Part print with two shaded views. Sizes in mm from the minimum x, y, z corner. A direction names the side the tool comes from. Give positions to 0.01 mm unless a question says otherwise; leave off trailing zeros. Write each loop counter-clockwise with the first axis right and the second up, starting at its lowest first coordinate (ties: lowest second). Pieces come first, ordered by that corner, then holes. Notation, with made-up numbers: (66, 7) - (103, 7) arc R26 cw to (103, 23) - close; hole circle Ø3 at (1.25, 86). An arc over 180 degrees is marked (long way). One line per item, written item: value. Start each with the question number.
(1) Cut at D-D, the plane y = 9.25. List the corners of the cut face in (x, z).
(2) Cut at B-B, the plane z = 19. State how many separate pieces and enclosed holes the cut face has.
(3) Cut at A-A, the plane x = 3.6. List the corners of the cut face in (y, z).
(4) Probe L1, parallel to Z at x = 21, y = 10; L2, parallel to Y at x = 29.6, z = 15; L3, parallel to X at y = 3, z = 11.75. List the from-to ranges inside material, lowest first.
(5) Cut at C-C, the plane y = 3.5. List the corners of the cut face in (x, z), and give its area (3 significant figures).
(6) Drop flat-ended pins along their axis: P1, Ø4.5, axis at x = 16.5, y = 12, coming from the -Z side; P2, Ø1, axis at x = 18, z = 9, coming from the +Y side (1 decimal); P3, Ø12.5, axis at x = 23, z = 10.5, coming from the +Y side. Give the stop position or say it passes through.
(7) 3-axis set-ups, long thin cutter, end or side, ignore diameter. For the marked faces 1 and 2: which of +Z, -Z, +X, -X, +Y, -Y reach the whole face in a straight line?
(8) Mould opens along Z. For the marked faces 3, 4 and 5 say: pulls with the +Z half, pulls with the -Z half, needs draft (parallel to the pull), parting line crosses it, or undercut.
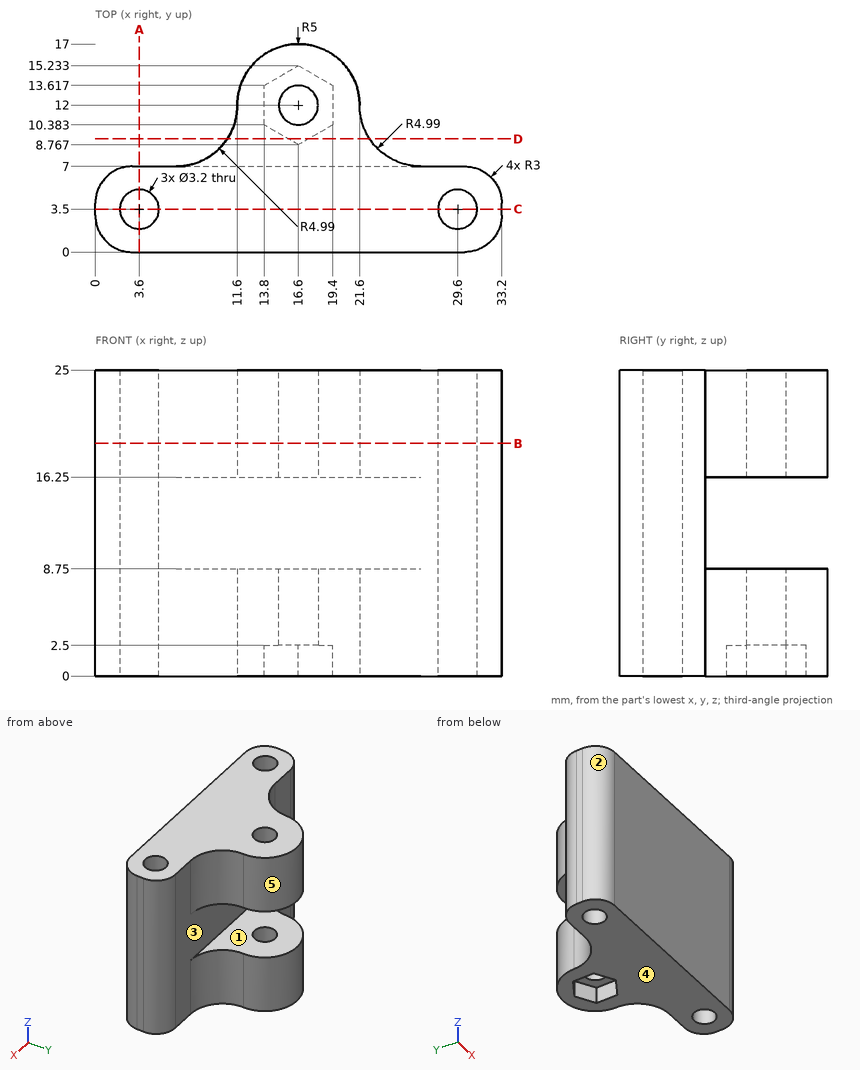
Answers follow:
1. outline: (10.78, 0) - (15.76, 0) - (15.76, 2.5) - (17.44, 2.5) - (17.44, 0) - (22.42, 0) - (22.42, 8.75) - (10.78, 8.75) - close; (10.78, 16.25) - (22.42, 16.25) - (22.42, 25) - (10.78, 25) - close
2. separate pieces: 1
2. enclosed holes: 3
3. outline: (0, 0) - (1.9, 0) - (1.9, 25) - (0, 25) - close; (5.1, 0) - (7, 0) - (7, 25) - (5.1, 25) - close
4. L1: z = 0 to 8.75, 16.25 to 25
4. L2: y = 0 to 1.9, 5.1 to 7
4. L3: x = 0 to 2.08, 5.12 to 28.08, 31.12 to 33.2
5. outline: (0, 0) - (2, 0) - (2, 25) - (0, 25) - close; (5.2, 0) - (28, 0) - (28, 25) - (5.2, 25) - close; (31.2, 0) - (33.2, 0) - (33.2, 25) - (31.2, 25) - close
5. area: 670 mm²
6. P1: stops at z = 2.5
6. P2: stops at y = 16.9
6. P3: stops at y = 16.98
7. face 1: +X, -X, +Y
7. face 2: +Z, -Z, -X, -Y
8. face 3: undercut
8. face 4: pulls with the -Z half
8. face 5: needs draft
